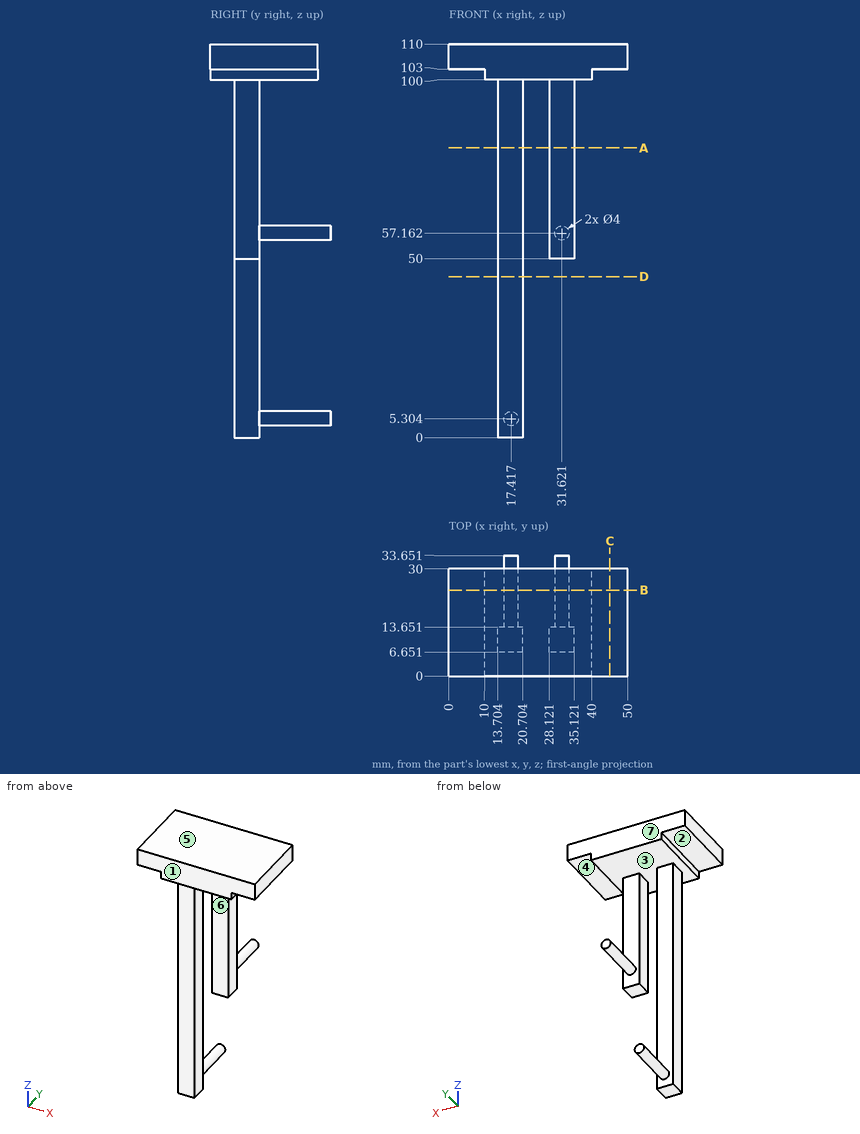
Input: dimensioned drawing with shaded views. Units: mm. Origin: part minimum x, y, z. A direction names the side the tool comes from. Give positions to 0.01 mm unless a question says otherwise; leave off trailing zeros. Order: outer loops, then holes, each group sorted by start corner. A loop starts at its lowest first (then second) coordinate and runs counter-clockwise, first axis right, second up. Notation, with made-up numbers: (-34, 61.25) -> (8, 61.25) arc R25 cw to (8, 95.25) -> close; hole circle Ø8 at (-39, 67). An arc over 180 degrees is marked (long way). Use a Markdown table: item, result.
1) Reachability of the marked faces 4, 5, 6 and 7 from +Z, -Z, +X, -X, +Y, -Y: full face, straight path, thin tool, end or side. Return the list, or none.
Answer list:
| item | result |
|---|---|
| face 4 | -Z, +X, +Y, -Y |
| face 5 | +Z, +X, -X, +Y, -Y |
| face 6 | -Z, +X, -X, -Y |
| face 7 | +Z, +X, -X, +Y |
2) Section query D-D, the plane z = 45. Return the cut outline in (x, y), then the cut area to 3 significant figures.
Answer list:
| item | result |
|---|---|
| outline | (13.7, 6.65) -> (20.7, 6.65) -> (20.7, 13.65) -> (13.7, 13.65) -> close |
| area | 49.0 mm² |
3) Section query A-A, the plane z = 81. Return the cut outline in (x, y), then the cut area to 3 significant figures.
Answer list:
| item | result |
|---|---|
| outline | (13.7, 6.65) -> (20.7, 6.65) -> (20.7, 13.65) -> (13.7, 13.65) -> close; (28.12, 6.65) -> (35.12, 6.65) -> (35.12, 13.65) -> (28.12, 13.65) -> close |
| area | 98.0 mm² |
4) Section query C-C, the plane x = 45. Return the cut outline in (y, z), then the cut area to 3 significant figures.
Answer list:
| item | result |
|---|---|
| outline | (0, 103) -> (30, 103) -> (30, 110) -> (0, 110) -> close |
| area | 210 mm² |
5) Mould query, pull axis Z, two halves, no side actions, for the marked faces 1, 2 and 3. Classes: +Z half, -Z half, draft (parallel to the pull), parting line (faces both ways), or undercut.
Answer list:
| item | result |
|---|---|
| face 1 | draft |
| face 2 | -Z half |
| face 3 | undercut |
6) Ray query, line 1 along X through (y, z) = (9, 72); line 2 along Z through (x, y) = (22, 5.5); line 3 along X through (y, z) = (8, 32). Return the intervals inside material, ascending. Write a range as [from, to].
Answer list:
| item | result |
|---|---|
| line 1 | [13.7, 20.7], [28.12, 35.12] |
| line 2 | [100, 110] |
| line 3 | [13.7, 20.7] |
7) Section query B-B, the plane y = 24. Return the cut outline in (x, z).
Answer list:
| item | result |
|---|---|
| outline | (0, 103) -> (10, 103) -> (10, 100) -> (40, 100) -> (40, 103) -> (50, 103) -> (50, 110) -> (0, 110) -> close; circle Ø4 at (17.42, 5.3); circle Ø4 at (31.62, 57.16) |
8) Contact query for flat-ended pins moving along their axis: P1, Ø0.9, axis at y = 8, z = 102, coming from the -X side; P2, Ø3.5, axis at y = 12, z = 82, coming from the -X side; P3, Ø3, axis at y = 5.5, z = 52.5, coming from the +X side. Output: stop coordinate, or through.
Answer list:
| item | result |
|---|---|
| P1 | x = 10 |
| P2 | x = 13.7 |
| P3 | x = 35.12 |
